The listing builds one solid part. Answer for the finished solid, in the listing's coordinates (mm). A direction names the side the tool comes from. Coordinates: 2 decimals unless noted, no trailing zeros. Loops run counter-clockwise (first coordinate to the right, second up) from the corner with the lowest first, then second, coordinate; pieces in that order, holes last. Notation, with made-up numbers: M 88,31 L 145,31 A15 ccw 145,47 Z; hole C 2,40 d7. An arc over 180 degrees is marked long. Answer as a JSON object with one key per item and string values. Group by question number.
1. A cutting plane is placed at C-C on y = 15. Give the vertices of the cut face in (x, z), and give its area (3 significant figures).
2. Straight lines are drawn through the part: L1, parallel to X at y = 17, z = 1; L2, parallel to Y at x = 28.5, z = -4. For each, find the intervals that lie inside material, in ascending order.
3. A cutting plane is placed at B-B on z = 3.5. Give the vertices of the cut face in (x, y), and give its area (3 significant figures).
4. A cutting plane is placed at A-A on x = 27.5. Give the vertices of the cut face in (y, z).
5. Given pin 1 (9 mm diameter, centred on x = -28.5, z = -2, fed in from +Y); pin 2 (3 mm diameter, centred on x = -27.5, y = 1.5, fed in from +Z); pin 3 (4.5 mm diameter, centred on x = 28.5, y = 2, fed in from +Z), each flat-ended and moving along its own axis, determine where each tip first touches the part or whether it passes through.
6. For faces 5 (the face through (24, 4, -1)), 6 (the face through (-24, 4, -1)), 7 (the face through (27.18, 1.97, 5.74)), determine the directions among +Z, -Z, +X, -X, +Y, -Y from which every point of the face is accessible in a straight line to the end or side of a thin tool.
7. A cutting plane is placed at D-D on z = 0. Give the vertices of the cut face in (x, y).
8. Determine the mould class of faces 1 (the face through (-29, 2, -2)), 2 (the face through (-27.18, 1.97, 5.74)), 3 (the face through (-23, 9, 0)), 4 (the face through (-29, 2, 2)) for opening direction Z: released by +Z, released by -Z, zero draft, split by the parting line, or undercut.
from build123d import *

# Parameters (mm, degrees)
SKETCH1_W           = 23
SKETCH1_H           = 32
BOSS_EXTRUDE1_DEPTH = 18
BOSS_EXTRUDE2_DEPTH = 4


with BuildPart() as part:
    # Sketch1 → Boss-Extrude1 (new body)
    with BuildSketch(Plane(origin=(0, 0, 0), x_dir=(1, 0, 0), z_dir=(0, 1, 0))):
        with Locations((-11.5, 0)):
            Rectangle(SKETCH1_W, SKETCH1_H)
    boss_extrude1 = extrude(amount=BOSS_EXTRUDE1_DEPTH)

    # Sketch2 → Boss-Extrude2 (add)
    with BuildSketch(Plane.XZ):
        with BuildLine():
            Line((-31.25, -5), (-31.25, -2))
            Line((-31.25, -2), (-26, -2))
            ThreePointArc((-26, -2), (-24, 0), (-26, 2))
            Line((-26, 2), (-31.25, 2))
            Line((-31.25, 2), (-31.25, 5))
            Line((-31.25, 5), (-23, 6.5))
            Line((-23, 6.5), (-23, -6.5))
            Line((-23, -6.5), (-31.25, -5))
        make_face()
    boss_extrude2 = extrude(amount=-BOSS_EXTRUDE2_DEPTH)

    # Mirror1: Boss-Extrude1, Boss-Extrude2 across plane
    add(boss_extrude1.mirror(Plane(origin=(0, 18, 16), x_dir=(0, 0, 1), z_dir=(-1, 0, 0))))
    add(boss_extrude2.mirror(Plane(origin=(0, 18, 16), x_dir=(0, 0, 1), z_dir=(-1, 0, 0))))


solid = part.part
From the geometry:
{
 "1": {"outline": "M -23,-16 L 23,-16 L 23,16 L -23,16 Z", "area": "1,470 mm²"},
 "2": {"L1": "x = -23 to 23", "L2": "y = 0 to 4"},
 "3": {"outline": "M -31.25,0 L 31.25,0 L 31.25,4 L 23,4 L 23,18 L -23,18 L -23,4 L -31.25,4 Z", "area": "894 mm²"},
 "4": {"outline": "M 0,-5.68 L 4,-5.68 L 4,-2 L 0,-2 Z; M 0,2 L 4,2 L 4,5.68 L 0,5.68 Z"},
 "5": {"pin 1": "stops at y = 4", "pin 2": "stops at z = 5.95", "pin 3": "stops at z = 5.91"},
 "6": {"face 5": "+Z, -Z, +X, +Y", "face 6": "+Z, -Z, -X, +Y", "face 7": "+Z, +X, +Y, -Y"},
 "7": {"outline": "M -24,0 L 24,0 L 24,4 L 23,4 L 23,18 L -23,18 L -23,4 L -24,4 Z"},
 "8": {"face 1": "undercut", "face 2": "released by +Z", "face 3": "zero draft", "face 4": "undercut"}
}
